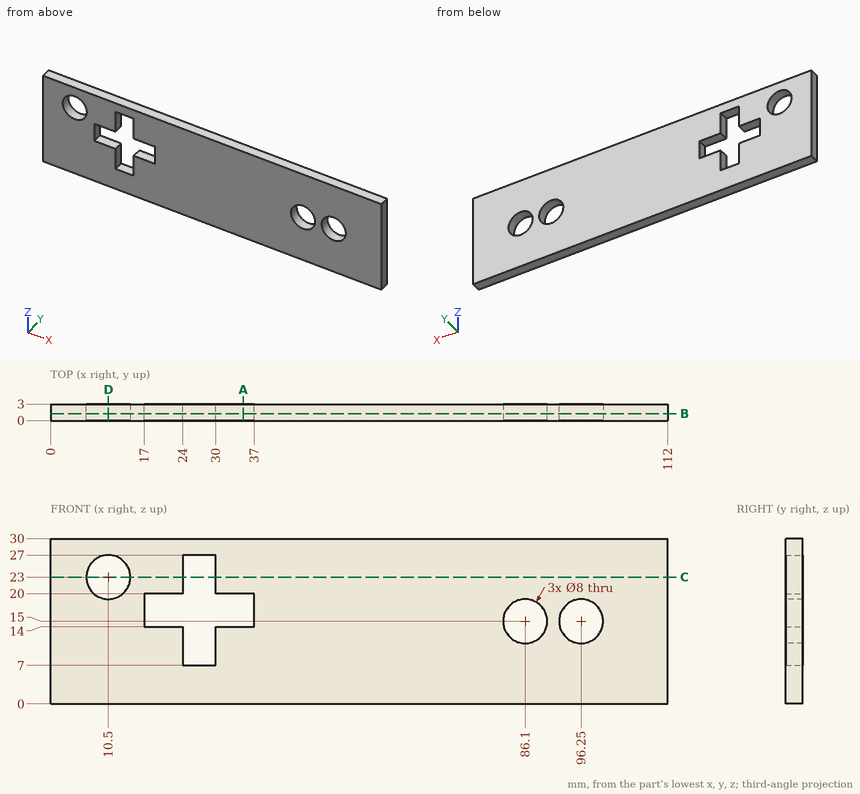
Design review of the part shown in the three views and the two pictorial views. Dimensions are in mm from the part's minimum x, y and z. Give positions to 0.01 mm unless a question says otherwise; leave off trailing zeros. Write each loop counter-clockwise with the first axis right and the second up, starting at its lowest first coordinate (ties: lowest second). Pieces come first, ordered by that corner, then holes. Notation, with made-up numbers: (23.5, -9.75) - (73.5, -9.75) arc R29 ccw to (73.5, 15.25) - close; hole circle Ø8 at (-2.5, 14.5). An arc over 180 degrees is marked (long way). Return JSON: item names as keys, results as strings. Group by question number.
(1) We need section A-A, the plane x = 35. Give the boundary of the cut face in (y, z).
(2) To check wall thickness, follow probe 1 along Z at (x, y) = (86.1, 1.4); probe 2 along Z at (x, y) = (10.5, 2.25); probe 3 along X at (y, z) = (0.85, 25.5). State the ranges of each line that lie inside material, in increasing order.
(3) We need section C-C, the plane z = 23. Give the boundary of the cut face in (x, y).
(4) We need section B-B, the plane y = 1.25. Give the boundary of the cut face in (x, z), then the cut area to 3 significant figures.
(5) We need section D-D, the plane x = 10.5. Give the boundary of the cut face in (y, z).
Reported:
{
 "1": {"outline": "(0, 0) - (3, 0) - (3, 14) - (0, 14) - close; (0, 20) - (3, 20) - (3, 30) - (0, 30) - close"},
 "2": {"probe 1": "z = 0 to 11, 19 to 30", "probe 2": "z = 0 to 19, 27 to 30", "probe 3": "x = 0 to 7.38, 13.62 to 24, 30 to 112"},
 "3": {"outline": "(0, 0) - (6.5, 0) - (6.5, 3) - (0, 3) - close; (14.5, 0) - (24, 0) - (24, 3) - (14.5, 3) - close; (30, 0) - (112, 0) - (112, 3) - (30, 3) - close"},
 "4": {"outline": "(0, 0) - (112, 0) - (112, 30) - (0, 30) - close; hole circle Ø8 at (10.5, 23); hole (17, 14) - (24, 14) - (24, 7) - (30, 7) - (30, 14) - (37, 14) - (37, 20) - (30, 20) - (30, 27) - (24, 27) - (24, 20) - (17, 20) - close; hole circle Ø8 at (86.1, 15); hole circle Ø8 at (96.25, 15)", "area": "3,010 mm2"},
 "5": {"outline": "(0, 0) - (3, 0) - (3, 19) - (0, 19) - close; (0, 27) - (3, 27) - (3, 30) - (0, 30) - close"}
}
